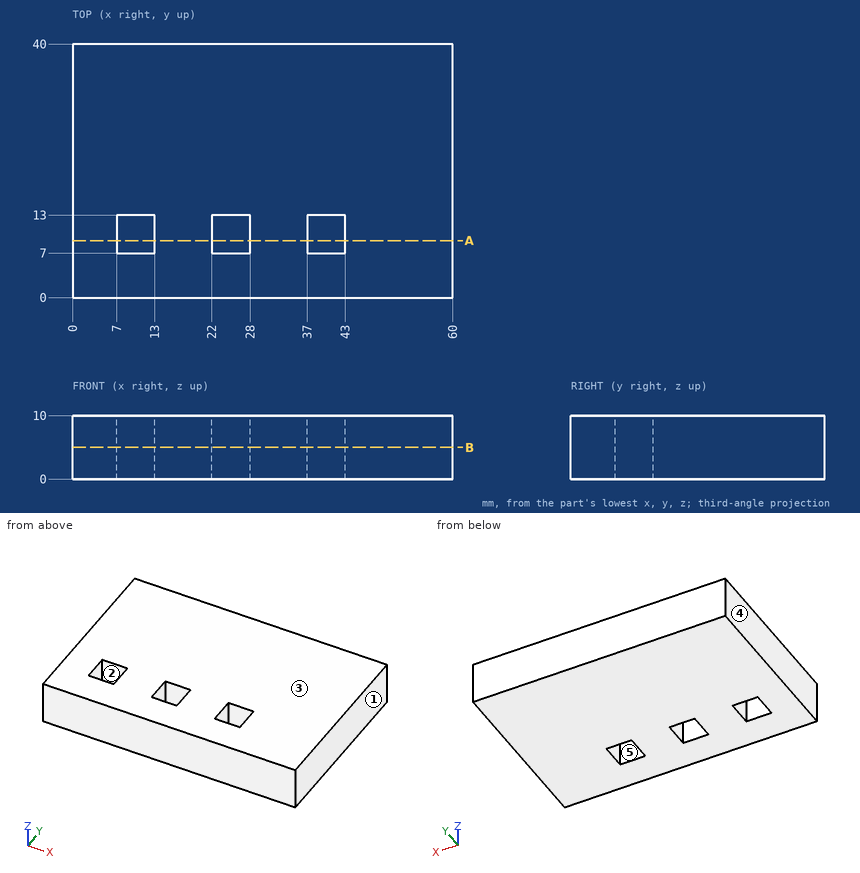
Here's the drawing with two shaded views (mm, measured from the low corner). I have some questions. A direction names the side the tool comes from. Give positions to 0.01 mm unless a question says otherwise; leave off trailing zeros. Loops run counter-clockwise (first coordinate to the right, second up) from the corner with the lowest first, then second, coordinate; pieces in that order, holes last. Notation, with made-up numbers: M 54,27 L 62,27 A28 cw 62,55 Z; hole C 67.5,0.5 d4. An arc over 180 degrees is marked long. One line per item, written item: value.
(1) Which directions (+Z, -Z, +X, -X, +Y, -Y) give clear straight access to the entire face, cutting with the end or side of a thin tool? Please do the marked faces 1 and 2.
Returned:
face 1: +Z, -Z, +X, +Y, -Y
face 2: +Z, -Z
(2) We'd pull the mould along X, two halves only. Please class the marked faces 3, 4 and 5: released by +X, released by -X, zero draft, split by the parting line, or undercut.
Returned:
face 3: zero draft
face 4: released by -X
face 5: undercut
(3) I need wall thicknesses on line 1 (X direction, y = 8.5, z = 5.75); line 2 (Y direction, x = 40.5, z = 7.75). Which ranges of each line are inside material? Lowest first, please.
Returned:
line 1: 0 to 7, 13 to 22, 28 to 37, 43 to 60
line 2: 0 to 7, 13 to 40
(4) Suppose I cut it at B-B on z = 5. List the corners of the cut face in (x, y) for me, plus the area to 3 significant figures.
Returned:
outline: M 0,0 L 60,0 L 60,40 L 0,40 Z; hole M 7,7 L 13,7 L 13,13 L 7,13 Z; hole M 22,7 L 28,7 L 28,13 L 22,13 Z; hole M 37,7 L 43,7 L 43,13 L 37,13 Z
area: 2,290 mm^2
(5) Suppose I cut it at A-A on y = 9. List the corners of the cut face in (x, z) for me, plus the area to 3 significant figures.
Returned:
outline: M 0,0 L 7,0 L 7,10 L 0,10 Z; M 13,0 L 22,0 L 22,10 L 13,10 Z; M 28,0 L 37,0 L 37,10 L 28,10 Z; M 43,0 L 60,0 L 60,10 L 43,10 Z
area: 420 mm^2
